CAD build for the part. Positions are in the model's coordinates, mm. A direction names the side the tool comes from. Coordinates: 2 decimals unless noted, no trailing zeros. Order: outer loops, then holes, each group sorted by start corner. A loop starts at its lowest first (then second) coordinate and runs counter-clockwise, first axis right, second up. Notation, with made-up numbers: M -34,17.5 L 13,17.5 A19 cw 13,27.5 Z; hole C 62.25,0.5 d10. An arc over 180 degrees is marked long. Write item = value, one per line.
from build123d import *

# Parameters (mm, degrees)
SKETCH1_W           = 127
SKETCH1_H           = 57.15
BOSS_EXTRUDE1_DEPTH = 9.525
SKETCH2_W           = 127
SKETCH2_H           = 127
BOSS_EXTRUDE3_DEPTH = 9.525
SKETCH3_R           = 10.16
CUT_EXTRUDE1_DEPTH  = 5.0038


with BuildPart() as part:
    # Sketch1 → Boss-Extrude1 (new body)
    with BuildSketch(Plane.XY):
        with Locations((63.5, 28.575)):
            Rectangle(SKETCH1_W, SKETCH1_H)
    extrude(amount=BOSS_EXTRUDE1_DEPTH)

    # Sketch2 → Boss-Extrude3 (add)
    with BuildSketch(Plane(origin=(0, 0, 0), x_dir=(1, 0, 0), z_dir=(0, 1, 0))):
        with Locations((63.5, 58.4962)):
            Rectangle(SKETCH2_W, SKETCH2_H)
    extrude(amount=BOSS_EXTRUDE3_DEPTH)

    # Sketch3 → Cut-Extrude1 (cut)
    with BuildSketch(Plane(origin=(0, 0, 0), x_dir=(1, 0, 0), z_dir=(0, 1, 0))):
        with Locations((63.5, 36.322)):
            Circle(SKETCH3_R)
    extrude(amount=CUT_EXTRUDE1_DEPTH, mode=Mode.SUBTRACT)


solid = part.part
(1) Slice it at C-C, the plane y = 16. Write the cut outline in (x, z) (3 decimals).
Evaluation:
outline = M 0,0 L 127,0 L 127,9.525 L 0,9.525 Z
(2) Slice it at B-B, the plane z = -38. Write the cut outline in (x, y) (3 decimals).
Evaluation:
outline = M 0,0 L 53.48,0 L 53.48,5.004 L 73.52,5.004 L 73.52,0 L 127,0 L 127,9.525 L 0,9.525 Z
(3) Slice it at A-A, the plane x = 63.5. Write the cut outline in (y, z) (3 decimals), then the cut area to 3 significant figures.
Evaluation:
outline = M 0,-121.996 L 9.525,-121.996 L 9.525,0 L 57.15,0 L 57.15,9.525 L 0,9.525 L 0,-26.162 L 5.004,-26.162 L 5.004,-46.482 L 0,-46.482 Z
area = 1,600 mm²
(4) Pull direction X, two halves, no side cores. Call faces 4 (the face through (63, 9.525, -62)), 5 (the face through (63, 5.004, -36)), 6 (the face through (127, 9, -42)): +X half, -X half, draft (parallel to the pull), parting line (faces both ways), or undercut.
Evaluation:
face_4 = draft
face_5 = undercut
face_6 = +X half
(5) Pin check, flat tips, straight feed: pin 1 Ø12 at (x, z) = (18.5, -59) entering from +Y (3 decimals); pin 2 Ø6 at (x, z) = (63.5, -38) entering from -Y. Stop position of each tip, or through.
Evaluation:
pin_1 = 9.525
pin_2 = 5
(6) Tool access for faces 1 (the face through (0, 9, -42)), 2 (the face through (63, 34, 0)), 3 (the face through (72.885, 2.467, -32.431)): list every direction of +Z, -Z, +X, -X, +Y, -Y with a clear straight run to the whole face (end or side of a thin tool).
Evaluation:
face_1 = +Z, -Z, -X, +Y, -Y
face_2 = -Z, +X, -X, +Y
face_3 = -Y
(7) Wall check: line 1 (Z direction, x = 63.5, y = 2.8) (3 decimals); line 2 (Y direction, x = 51.5, z = -71) (3 decimals). Give the ranges that are in metal, low to high. Write a range as from..to.
Evaluation:
line_1 = -121.996..-46.482, -26.162..9.525
line_2 = 0..9.525
